The listing builds one solid part. Answer for the finished solid, in the listing's coordinates (mm). A direction names the side the tool comes from. Give positions to 0.01 mm unless a question says otherwise; leave off trailing zeros. Write each loop counter-clockwise with the first axis right and the second up, starting at its lowest first coordinate (ties: lowest second). Pieces come first, ordered by that corner, then holes. Notation, with made-up numbers: (-17.5, 35.5) - (36.5, 35.5) arc R5 ccw to (36.5, 41.5) - close; hole circle Ø9 at (59, 41.25). An arc over 180 degrees is marked (long way). Use a Markdown table: item, result. Add a question column.
from build123d import *

# Parameters (mm, degrees)
ESBO_O1_W                = 60
ESBO_O1_H                = 60
BASE_DEPTH               = 2
ESBO_O3_W                = 24.3
ESBO_O3_H                = 24.3
ESBO_O3_W_2              = 18.3
ESBO_O3_H_2              = 18.3
ENCAIXES_DA_ARVORE_DEPTH = 5.5
ESBO_O4_W                = 60
ESBO_O4_H                = 60
ESBO_O4_W_2              = 52
ESBO_O4_H_2              = 52
PAREDES_DEPTH            = 8
ESBO_O5_W                = 7
ESBO_O5_H                = 7
CORTE_DOS_ENCAIXE_DEPTH  = 5.5
ESBO_O6_W                = 56
ESBO_O6_H                = 56
ESBO_O6_W_2              = 52
ESBO_O6_H_2              = 52
CORTE_EXTRUS_O2_DEPTH    = 2.5
FILETE5_R                = 1.5
FILETE6_R                = 3
ESBO_O7_W                = 10
ESBO_O7_H                = 5.5
CORTE_EXTRUS_O3_DEPTH    = 65.311740763
CHANFRO2_SIZE            = 2
FILETE19_R               = 1
FILETE20_R               = 5


with BuildPart() as part:
    # Esboço1 → Base (new body)
    with BuildSketch(Plane(origin=(0, 0, 0), x_dir=(1, 0, 0), z_dir=(0, 1, 0))):
        Rectangle(ESBO_O1_W, ESBO_O1_H)
    extrude(amount=BASE_DEPTH)

    # Esboço3 → Encaixes da Arvore (add)
    with BuildSketch(Plane(origin=(0, 2, 0), x_dir=(1, 0, 0), z_dir=(0, 1, 0))):
        Rectangle(ESBO_O3_W, ESBO_O3_H)
        Rectangle(ESBO_O3_W_2, ESBO_O3_H_2, mode=Mode.SUBTRACT)
    extrude(amount=ENCAIXES_DA_ARVORE_DEPTH)

    # Esboço4 → Paredes (add)
    with BuildSketch(Plane(origin=(0, 2, 0), x_dir=(1, 0, 0), z_dir=(0, 1, 0))):
        Rectangle(ESBO_O4_W, ESBO_O4_H)
        Rectangle(ESBO_O4_W_2, ESBO_O4_H_2, mode=Mode.SUBTRACT)
    extrude(amount=PAREDES_DEPTH)

    # Esboço5 → Corte dos Encaixe (cut)
    with BuildSketch(Plane(origin=(0, 7.5, 0), x_dir=(1, 0, 0), z_dir=(0, 1, 0))):
        with Locations((8.65, 8.65)):
            Rectangle(ESBO_O5_W, ESBO_O5_H)
        with Locations((-8.65, 8.65)):
            Rectangle(ESBO_O5_W, ESBO_O5_H)
        with Locations((8.65, -8.65)):
            Rectangle(ESBO_O5_W, ESBO_O5_H)
        with Locations((-8.65, -8.65)):
            Rectangle(ESBO_O5_W, ESBO_O5_H)
    extrude(amount=-CORTE_DOS_ENCAIXE_DEPTH, mode=Mode.SUBTRACT)

    # Esboço6 → Corte-extrusão2 (cut)
    with BuildSketch(Plane(origin=(0, 10, 0), x_dir=(1, 0, 0), z_dir=(0, 1, 0))):
        Rectangle(ESBO_O6_W, ESBO_O6_H)
        Rectangle(ESBO_O6_W_2, ESBO_O6_H_2, mode=Mode.SUBTRACT)
    extrude(amount=-CORTE_EXTRUS_O2_DEPTH, mode=Mode.SUBTRACT)

    # Filete5
    filete5_edges = [part.edges().sort_by_distance(p)[0] for p in [
        (26, 4.75, 26),
        (26, 4.75, -26),
        (-26, 4.75, 26),
        (-26, 4.75, -26),
    ]]
    fillet(filete5_edges, radius=FILETE5_R)

    # Filete6
    filete6_edges = [part.edges().sort_by_distance(p)[0] for p in [
        (-28, 8.75, 28),
        (-28, 8.75, -28),
        (28, 8.75, -28),
        (28, 8.75, 28),
    ]]
    fillet(filete6_edges, radius=FILETE6_R)

    # Esboço7 → Corte-extrusão3 (cut, through all)
    with BuildSketch(Plane.ZY.offset(-26)):
        with Locations((-17.5, 4.75)):
            Rectangle(ESBO_O7_W, ESBO_O7_H)
    extrude(amount=-CORTE_EXTRUS_O3_DEPTH, mode=Mode.SUBTRACT)

    # Chanfro2
    chanfro2_edges = [part.edges().sort_by_distance(p)[0] for p in [
        (-12.15, 2, 0),
        (0, 2, -12.15),
        (12.15, 2, 0),
        (0, 2, 12.15),
    ]]
    chamfer(chanfro2_edges, length=CHANFRO2_SIZE)

    # Filete19
    filete19_edges = [part.edges().sort_by_distance(p)[0] for p in [
        (9.15, 4.75, -5.15),
        (5.15, 4.75, -9.15),
        (5.15, 4.75, 9.15),
        (9.15, 4.75, 5.15),
        (-9.15, 4.75, 5.15),
        (-5.15, 4.75, 9.15),
        (-5.15, 4.75, -9.15),
        (-9.15, 4.75, -5.15),
    ]]
    fillet(filete19_edges, radius=FILETE19_R)

    # Filete20
    filete20_edges = [part.edges().sort_by_distance(p)[0] for p in [
        (30, 5, 30),
        (-30, 5, 30),
        (-30, 5, -30),
        (30, 5, -30),
    ]]
    fillet(filete20_edges, radius=FILETE20_R)


solid = part.part
1. Which of the six approach directions +Z, -Z, +X, -X, +Y, -Y give full straight-line access (tool end or side, diameter ignored) to faces 1 (the flat face through (29, 7.5, -18)), 2 (the flat face through (-30, 5, 0)), 3 (the flat face through (0, 5, 26))?
2. The part is cut by section B-B (x = 6.5). Give the vertices of the cut face in (y, z), and give its area (3 significant figures).
3. Consider L1, parallel to X at y = 5.25, z = -2.5; L2, parallel to Z at x = -20.5, y = 6.75. Determine where each line is inside the solid, lowest interval first. Write a range as [from, to].
4. The part is cut by section A-A (z = -20). Give the vertices of the cut face in (x, y), and give its area (3 significant figures).
5. Given P1, Ø3.5, axis at x = 11.5, z = 2, coming from the +Y side; P2, Ø1.2, axis at x = 28.5, y = 4, coming from the +Z side; P3, Ø2, axis at x = -23, z = -11.5, coming from the -Y side, each flat-ended and moving along its own axis, determine where each tip first touches the part or whether it passes through.
6. The part is cut by section C-C (y = 9.25). Give the vertices of the cut face in (x, z).
7. For a pull along X with two mould halves and no side action, classify faces 4 (the flat face through (0, 5, 9.15)), 5 (the flat face through (0, 0, 0)), 6 (the cylindrical face through (-28, 5, 29)) as released by +X, released by -X, zero draft, split by the parting line, or undercut.
8. The part is cut by section D-D (z = -1.5). Give the vertices of the cut face in (x, y), and give its area (3 significant figures).
Check values:
| question | item | result |
|---|---|---|
| 1 | face 1 | +X |
| 1 | face 2 | +Z, -Z, -X, +Y, -Y |
| 1 | face 3 | +Y |
| 2 | outline | (0, -30) - (10, -30) - (10, -28) - (7.5, -28) - (7.5, -26) - (2, -26) - (2, 26) - (7.5, 26) - (7.5, 28) - (10, 28) - (10, 30) - (0, 30) - close |
| 2 | area | 174 mm2 |
| 3 | L1 | x = [-30, -26], [-12.15, -9.15], [9.15, 12.15], [26, 30] |
| 3 | L2 | z = [-30, -26], [26, 30] |
| 4 | outline | (-30, 0) - (30, 0) - (30, 2) - (-26, 2) - (-26, 7.5) - (-28, 7.5) - (-28, 10) - (-30, 10) - close; (28, 7.5) - (30, 7.5) - (30, 10) - (28, 10) - close |
| 4 | area | 152 mm2 |
| 5 | P1 | stops at y = 7.5 |
| 5 | P2 | stops at z = 29.07 |
| 5 | P3 | stops at y = 0 |
| 6 | outline | (-30, -25) arc R5 ccw to (-25, -30) - (25, -30) arc R5 ccw to (30, -25) - (30, 25) arc R5 ccw to (25, 30) - (-25, 30) arc R5 ccw to (-30, 25) - close; hole (-28, -25) arc R3 ccw to (-25, -28) - (25, -28) arc R3 ccw to (28, -25) - (28, 25) arc R3 ccw to (25, 28) - (-25, 28) arc R3 ccw to (-28, 25) - close |
| 7 | face 4 | undercut |
| 7 | face 5 | zero draft |
| 7 | face 6 | released by -X |
| 8 | outline | (-30, 0) - (30, 0) - (30, 10) - (28, 10) - (28, 7.5) - (26, 7.5) - (26, 2) - (14.15, 2) - (12.15, 4) - (12.15, 7.5) - (9.15, 7.5) - (9.15, 2) - (-9.15, 2) - (-9.15, 7.5) - (-12.15, 7.5) - (-12.15, 4) - (-14.15, 2) - (-26, 2) - (-26, 7.5) - (-28, 7.5) - (-28, 10) - (-30, 10) - close |
| 8 | area | 211 mm2 |
